Autodesk Inventor part; units mm, degrees
ref_plane "작업 평면2" through (-79.061, -70.6061, -13.8) normal (0, 0, 1) x (1, 0, 0)
ref_plane "YZ Plane" through (0, 0, 0) normal (1, 0, 0) x (0, 1, 0)
ref_plane "XZ Plane" through (0, 0, 0) normal (0, 1, 0) x (-1, 0, 0)
ref_plane "작업 평면1" through (-9.061, -9.3, 6.3) normal (-1, 0, 0) x (0, 1, 0)
sketch "스케치1" plane through (-9.061, -9.3, 6.3) normal (-1, 0, 0) x (0, 1, 0)
  line L0 (39.3939, -39.95) -> (-0.6061, -39.95)
  line L1 (-0.6061, 0.55) -> (39.3939, 0.55)
  line L2 (-0.6061, -12.65) -> (-7.8061, -12.65)
  line L3 (-7.8061, -12.65) -> (-7.8061, -9.45)
  line L4 (-7.8061, -9.45) -> (-0.6061, -9.45)
  line L5 (19.3939, -39.95) -> (19.3939, 0.55) construction
  line L6 (39.3939, -12.65) -> (46.5939, -12.65)
  line L7 (46.5939, -12.65) -> (46.5939, -9.45)
  line L8 (46.5939, -9.45) -> (39.3939, -9.45)
  line L9 (-0.6061, -39.95) -> (-0.6061, -12.65)
  line L10 (-0.6061, -9.45) -> (-0.6061, 0.55)
  line L11 (39.3939, 0.55) -> (39.3939, -9.45)
  line L12 (39.3939, -12.65) -> (39.3939, -39.95)
  line L13 (-9.1061, 1.1) -> (47.8939, 1.1)
  line L14 (39.6939, 1.1) -> (39.6939, -9.15)
  line L15 (39.6939, -9.15) -> (46.8939, -9.15)
  line L16 (46.8939, -9.15) -> (46.8939, -12.95)
  line L17 (46.8939, -12.95) -> (39.6939, -12.95)
  line L18 (39.6939, -12.95) -> (39.6939, -40.25)
  line L19 (39.6939, -40.25) -> (-0.9061, -40.25)
  line L20 (-0.9061, -40.25) -> (-0.9061, -12.95)
  line L21 (-0.9061, -12.95) -> (-8.1061, -12.95)
  line L22 (-8.1061, -12.95) -> (-8.1061, -9.15)
  line L23 (-8.1061, -9.15) -> (-0.9061, -9.15)
  line L24 (-0.9061, -9.15) -> (-0.9061, 1.1)
  line L25 (47.8939, 2.4305) -> (-9.1061, 2.4305)
  line L26 (-9.1061, 2.4305) -> (-9.1061, -41.8305)
  line L27 (-9.1061, -41.8305) -> (47.8939, -41.8305)
  line L28 (47.8939, -41.8305) -> (47.8939, 2.4305)
  line L29 (39.3939, -19.7) -> (-0.6061, -19.7) construction
  line L30 (39.6939, -26.25) -> (39.6939, -30.25)
  line L31 (-0.8061, 6.3) -> (19.1939, 6.3)
  line L32 (7.6194, 1.8) -> (13.6194, 1.8)
  line L33 (7.6194, 1.8) -> (13.6194, 1.8)
  line L34 (7.6194, 1.8) -> (13.6194, 1.8)
  line L35 (-0.9061, -31.1) -> (-4.9061, -31.1)
  line L36 (-4.9061, -31.1) -> (-4.9061, -36.1)
  line L37 (-4.9061, -36.1) -> (-0.9061, -36.1)
  line L38 (6.1939, 1.8) -> (12.1939, 1.8)
  point P0 (19.3939, -19.7)
  point P1 (9.1939, 6.3)
  dimension "d0" = 40.5
  dimension "d1" = 40
  dimension "d2" = 3.2
  dimension "d3" = 27.2
  dimension "d6" = 27.3
  dimension "d8" = 0.3
  dimension "d9" = 20.25
  dimension "d23" = 9.8
  dimension "d24" = 26
  dimension "d26" = 5
  dimension "d27" = 4
  dimension "d28" = 4.15
extrude "돌출1" add sketch "스케치1" against normal blind 22 contours L13 L24 L23 L22 L21 L20 L35 L36 L37 L19 L18 L17 L16 L15 L14 L28 L27 L26 | L20 L37 L36 L35
sketch "스케치4" plane through (12.939, -9.3, 6.3) normal (1, 0, 0) x (0, 0, -1)
  line L0 (-12.95, -0.9061) -> (-40.25, -0.9061)
  line L1 (-31.1, -0.9061) -> (-31.1, -4.9061)
  line L2 (-31.1, -4.9061) -> (-36.1, -4.9061)
  line L3 (-36.1, -4.9061) -> (-36.1, -0.9061)
  line L4 (-40.25, -0.9061) -> (-12.95, -0.9061)
  line L5 (-41.8305, -9.1061) -> (1.1, -9.1061)
  line L6 (-31.1, -4.9061) -> (-31.1, -9.1061)
  line L7 (-36.1, -4.9061) -> (-36.1, -9.1061)
  point P0 (6.3, 9.3)
extrude "돌출4" cut sketch "스케치4" against normal blind 22
sketch "스케치2" plane through (-9.061, -9.3, 6.3) normal (-1, 0, 0) x (0, 0, 1)
  line L0 (-1.1, -0.9061) -> (-1.1, -9.1061)
  line L1 (-1.1, -9.1061) -> (41.8305, -9.1061)
  line L2 (41.8305, -9.1061) -> (41.8305, 47.8939)
  line L3 (41.8305, 47.8939) -> (-1.1, 47.8939)
  line L4 (-1.1, 47.8939) -> (-1.1, 39.6939)
  line L5 (-1.1, 47.8939) -> (41.8305, 47.8939)
  line L6 (41.8305, 47.8939) -> (41.8305, -9.1061)
  line L7 (41.8305, -9.1061) -> (-1.1, -9.1061)
  line L8 (-1.1, -9.1061) -> (-1.1, 47.8939)
  point P0 (-6.3, 9.3)
  point P1 (-1.1, -0.9061)
extrude "돌출2" add sketch "스케치2" along normal blind 2
sketch "스케치3" plane through (12.939, -18.4061, 5.2) normal (0, 0, -1) x (-1, 0, 0)
  line L0 (22, 8.2) -> (0, 8.2)
  line L1 (22, 48.8) -> (0, 48.8)
  line L2 (22, 48.8) -> (22, 8.2)
  circle A0 centre (7.1, 4.2) radius 2
  line L3 (22, 28.5) -> (0, 28.5) construction
  line L4 (0, 8.2) -> (0, 48.8)
  circle A1 centre (7.1, 52.8) radius 2
  circle A2 centre (17, 4.2) radius 2
  circle A3 centre (17, 52.8) radius 2
  line L5 (12.05, 8.2) -> (12.05, 48.8)
  point P0 (12.939, 18.4061)
  dimension "d81" = 0
  dimension "d15" = 24.3
  dimension "d16" = 4
  dimension "d88" = 5
  dimension "d89" = 4.95
  dimension "d90" = 9.9
extrude "돌출3" cut sketch "스케치3" against normal blind 40 contours A0 | A1 | A2 | A3
sketch "스케치5" plane through (12.939, -9.3, 6.3) normal (1, 0, 0) x (0, 0, -1)
  line L0 (1.1, -9.1061) -> (1.1, -0.9061)
  line L1 (-9.15, -0.9061) -> (-9.15, -8.1061)
  line L2 (-36.1, -9.1061) -> (-36.1, -0.9061)
  line L3 (-36.1, -0.9061) -> (-40.25, -0.9061)
  line L4 (-40.25, -0.9061) -> (-40.25, 39.6939)
  line L5 (-40.25, 39.6939) -> (-12.95, 39.6939)
  line L6 (-12.95, 39.6939) -> (-12.95, 46.8939)
  line L7 (-12.95, 46.8939) -> (-9.15, 46.8939)
  line L8 (-9.15, 46.8939) -> (-9.15, 39.6939)
  line L9 (-9.15, 39.6939) -> (1.1, 39.6939)
  line L10 (1.1, 39.6939) -> (1.1, 47.8939)
  line L11 (1.1, 47.8939) -> (-41.8305, 47.8939)
  line L12 (-41.8305, 47.8939) -> (-41.8305, -9.1061)
  line L13 (-41.8305, -9.1061) -> (-36.1, -9.1061)
  line L14 (-12.95, -8.1061) -> (-9.15, -8.1061)
  line L15 (-9.15, -8.1061) -> (1.1, -8.1061)
  line L16 (1.1, -8.1061) -> (1.1, 46.8939)
  line L17 (1.1, 46.8939) -> (-9.15, 46.8939)
  line L18 (-9.15, 46.8939) -> (-9.15, -8.1061)
  point P0 (6.3, 9.3)
  point P1 (-9.15, -0.9061)
  point P2 (1.1, -8.1061)
  point P3 (1.1, -0.9061)
  point P4 (1.1, 39.6939)
  point P5 (-9.15, 46.8939)
extrude "돌출5" cut sketch "스케치5" against normal up to surface (22 mm away) contours L15 L1 L18 L9 L16 L0 | L9 L8 L17 L10
sketch "스케치12" plane through (12.939, -10.2061, 46.55) normal (0, 0, -1) x (-1, 0, 0)
  line L0 (22, 40.6) -> (0, 40.6)
  line L1 (0, 0) -> (0, 40.6)
  line L2 (22, 47.8) -> (0, 47.8)
  line L3 (1.5, 48.8) -> (1.5, -8.2)
  line L4 (0, -8.2) -> (24, -8.2)
  line L5 (0, -7.2) -> (0, 0)
  line L6 (0, -8.2) -> (0, -7.2)
  line L7 (0, 40.6) -> (0, 47.8)
  line L8 (0, 48.8) -> (24, 48.8)
  line L9 (0, 47.8) -> (0, 48.8)
  point P0 (12.939, 10.2061)
  point P1 (1.5, 40.6)
  dimension "d55" = 1.5
extrude "돌출12" add sketch "스케치12" along normal blind 41.35
sketch "스케치13" plane through (12.939, -18.4061, 5.2) normal (0, 0, -1) x (-1, 0, 0)
  line L0 (0, 0) -> (0, 57)
  line L1 (0, 0) -> (24, 0)
  line L2 (24, 57) -> (24, 0)
  line L3 (0, 57) -> (24, 57)
  line L4 (12, 0) -> (12, 57) construction
  line L5 (24, 28.5) -> (0, 28.5) construction
  line L6 (24, 8.2) -> (32, 8.2)
  line L7 (32, 8.2) -> (32, 16.2)
  line L8 (32, 16.2) -> (24, 16.2)
  line L9 (24, 16.2) -> (24, 8.2)
  line L10 (24, 40.8) -> (24, 48.8)
  line L11 (24, 0) -> (24, 57)
  line L12 (24, 48.8) -> (32, 48.8)
  line L13 (32, 48.8) -> (32, 40.8)
  line L14 (32, 40.8) -> (24, 40.8)
  line L15 (7, 57) -> (17, 57)
  line L16 (17, 57) -> (17, 62)
  line L17 (17, 62) -> (7, 62)
  line L18 (7, 62) -> (7, 57)
  point P0 (12.939, 18.4061)
  dimension "d70" = 8
  dimension "d71" = 8
  dimension "d72" = 8.2
  dimension "d73" = 10
  dimension "d74" = 5
extrude "돌출13" add sketch "스케치13" against normal blind 5 contours L18 L17 L16 L3 | L2 L8 L7 L6 | L2 L12 L13 L14
sketch "스케치14" plane through (-19.061, -10.2061, 5.2) normal (-1, 0, 0) x (0, 0, 1)
  line L0 (-34, 162.6) -> (-34, -37.7889)
  line L1 (-34, -37.7889) -> (-19, -37.7889)
  line L2 (-19, 162.6) -> (-19, -37.7889)
  line L3 (-34, 162.6) -> (-19, 162.6)
  line L4 (5, 0) -> (-19, 0)
  line L5 (-19, 0) -> (-19, 40.6)
  line L6 (-19, 40.6) -> (5, 40.6)
  line L7 (5, 40.6) -> (5, 0)
  line L8 (0, 32.6) -> (0, 40.6)
  line L9 (0, 32.6) -> (5, 32.6)
  line L10 (5, 40.6) -> (5, 32.6)
  line L11 (0, 40.6) -> (5, 40.6)
  point P0 (-5.2, 10.2061)
  point P1 (-19, 0)
extrude "돌출14" add sketch "스케치14" against normal blind 3 contours L6 L8 L9 L7 L4 L2 | L6 L7 L9 L8
sketch "스케치15" plane through (-19.061, -10.2061, -13.8) normal (0, 0, -1) x (-1, 0, 0)
  line L0 (0, 40.6) -> (0, 0)
  line L1 (0, 0) -> (10, 0)
  line L2 (10, 0) -> (10, 10)
  line L3 (10, 10) -> (0, 10)
  line L4 (0, 10) -> (0, 0)
  point P0 (-19.061, 10.2061)
  point P1 (0, 10)
  dimension "d66" = 10
  dimension "d67" = 10
extrude "돌출15" add sketch "스케치15" against normal blind 4
sketch "스케치16" plane through (12.939, -18.4061, 5.2) normal (0, 0, -1) x (-1, 0, 0)
  line L0 (17, 57) -> (17, 62)
  line L1 (17, 62) -> (7, 62)
  line L2 (7, 62) -> (7, 57)
  line L3 (7, 57) -> (17, 57)
  point P0 (12.939, 18.4061)
ref_plane "작업 평면2" through (-79.061, -70.6061, -13.8) normal (0, 0, 1) x (1, 0, 0)
extrude "돌출16" add sketch "스케치16" along normal up to surface (19 mm away)
sketch "스케치17" plane through (-4.061, 43.5939, 10.2) normal (0, 1, 0) x (1, 0, 0)
  line L0 (0, 0) -> (0, 24)
  line L1 (10, 24) -> (10, 0)
  line L2 (0, 24) -> (10, 24)
  line L3 (10, 20) -> (0, 20)
  point P0 (4.061, 10.2)
  dimension "d77" = 4
extrude "돌출17" add sketch "스케치17" along normal blind 10
sketch "스케치18" plane through (-19.061, -10.2061, -9.8) normal (0, 0, 1) x (1, 0, 0)
  circle A0 centre (-5, 5) radius 2
  point P0 (19.061, 10.2061)
  dimension "d80" = 4
extrude "돌출18" cut sketch "스케치18" against normal through all
ref_plane "작업 평면3" through (0.939, -9.3, 6.3) normal (1, 0, 0) x (0, 0, -1)
sketch "스케치19" plane through (-4.061, 43.5939, -9.8) normal (0, 0, 1) x (1, 0, 0)
  line L0 (0, 10) -> (10, 10)
  line L1 (0, 0) -> (0, 10)
  circle A0 centre (5, 5) radius 2
  point P0 (4.061, -43.5939)
  dimension "d83" = 4
  dimension "d84" = 5
  dimension "d85" = 5
extrude "돌출19" cut sketch "스케치19" against normal through all
mirror "미러1" about plane through (0.939, -9.3, 6.3) normal (1, 0, 0) of "돌출13", "돌출14", "돌출15", "돌출18"
ref_plane "작업 평면4" through (20.939, -10.2061, 10.2) normal (0, -1, 0) x (1, 0, 0)
split "분할1" plane through (20.939, -10.2061, 10.2) removes the side toward (0, -1, 0)
sketch "스케치20" plane through (12.939, 38.5939, 48.1305) normal (0, 1, 0) x (1, 0, 0)
  line L0 (-22, 1.5805) -> (-22, 42.9305)
  line L1 (-22, 23.6445) -> (-2, 23.6445)
  line L2 (-2, 23.6445) -> (-2, 8.6445)
  line L3 (-2, 8.6445) -> (-22, 8.6445)
  line L4 (-22, 8.6445) -> (-22, 23.6445)
  point P0 (-12.939, 48.1305)
  point P1 (-22, 8.6445)
  dimension "d91" = 15
  dimension "d92" = 20
extrude "돌출20" cut sketch "스케치20" against normal blind 10
properties part number "SAFRS-P-0012"
Source: CAD feature listing. Evaluate the final solid. Frame: model axes, mm. A direction names the side the tool comes from. Coordinates: 2 decimals unless noted, no trailing zeros. Loops run counter-clockwise (first coordinate to the right, second up) from the corner with the lowest first, then second, coordinate; pieces in that order, holes last. Notation, with made-up numbers: (89.25, 43) -> (113.25, 43) arc R7 ccw to (113.25, 50) -> close; hole circle Ø2 at (1, 51.5). An arc over 180 degrees is marked (long way). One line per item, written item: value. Start each with the question number.
Q1. Section query B-B, the plane z = -5. Return the cut outline in (x, y).
Q2. Mould query, pull axis X, two halves, no side actions, for faces 6 (the face through (-17, 30.394, 1)), 7 (the face through (24.031, -5.807, -11.772)), 8 (the face through (5.939, 43, -5)), 9 (the face through (-4.061, 43, -4)). Classes: pulls with the +X half, pulls with the -X half, needs draft (parallel to the pull), parting line crosses it, or undercut.
Q3. Section query C-C, the plane y = 1. Return the cut outline in (x, z).
Q4. Section query D-D, the plane z = 33.5. Return the cut outline in (x, y).
Q5. Contact query for flat-ended pins moving along their axis: P1, Ø1.5, axis at x = 10, z = 28, coming from the +Y side; P2, Ø12.5, axis at y = 20.5, z = 30, coming from the -X side; P3, Ø1.5, axis at y = 27.5, z = 32, coming from the +X side; P4, Ø10, axis at x = 4.5, z = 20, coming from the +Y side. Output: stop coordinate, or through.
Q6. Section query A-A, the plane x = 17. Return the cut outline in (y, z), and give its area (3 significant figures).
Q7. Line query: line 1 along X through (y, z) = (4, 33); line 2 along X through (y, z) = (5, 8); line 3 along X through (y, z) = (-6.5, 4.5). Output: solid intervals per line, ascending.
Q8. Set-up query: faces 1 (the face through (11.439, 14, 26)), 2 (the face through (-17, 10, 10.2)), 3 (the face through (1, 38.594, -4)), 4 (the face through (6, 34, 45.2)), 5 (the face through (1, 41, 10.2)). Return all of +Z, -Z, +X, -X, +Y, -Y with unobstructed straight access to the full face (end or side cutting, diameter ignored); none if empty.
Results:
1. outline: (-19.06, -10.21) -> (-16.06, -10.21) -> (-16.06, 30.39) -> (-19.06, 30.39) -> close; (-4.06, 38.59) -> (5.94, 38.59) -> (5.94, 43.59) -> (-4.06, 43.59) -> close; (17.94, -10.21) -> (20.94, -10.21) -> (20.94, 30.39) -> (17.94, 30.39) -> close
2. face 6: needs draft
2. face 7: undercut
2. face 8: pulls with the +X half
2. face 9: pulls with the -X half
3. outline: (-19.06, -13.8) -> (-16.06, -13.8) -> (-16.06, 10.2) -> (-19.06, 10.2) -> close; (-11.06, 5.2) -> (-9.06, 5.2) -> (-9.06, 46.55) -> (11.44, 46.55) -> (11.44, 5.2) -> (12.94, 5.2) -> (12.94, 48.13) -> (-11.06, 48.13) -> close; (17.94, -13.8) -> (20.94, -13.8) -> (20.94, 10.2) -> (17.94, 10.2) -> close
4. outline: (-11.06, -10.21) -> (-9.06, -10.21) -> (-9.06, 38.59) -> (-11.06, 38.59) -> close; (10.94, 30.39) -> (11.44, 30.39) -> (11.44, -10.21) -> (12.94, -10.21) -> (12.94, 38.59) -> (10.94, 38.59) -> close
5. P1: through
5. P2: x = -11.06
5. P3: x = 12.94
5. P4: y = 38.59
6. outline: (-10.21, 5.2) -> (-2.21, 5.2) -> (-2.21, 10.2) -> (-10.21, 10.2) -> close; (22.39, 5.2) -> (30.39, 5.2) -> (30.39, 10.2) -> (22.39, 10.2) -> close
6. area: 80.0 mm^2
7. line 1: -11.06 to -9.06, 11.44 to 12.94
7. line 2: -19.06 to -16.06, -11.06 to -9.06, 11.44 to 12.94, 17.94 to 20.94
7. line 3: -19.06 to -16.06, 17.94 to 20.94
8. face 1: -Z, -Y
8. face 2: +Z, -X, +Y, -Y
8. face 3: -Z, +X, -X, -Y
8. face 4: -Z
8. face 5: +Z, +X, -X, +Y
